Geometry: final body of the model. Coordinates: model frame, mm. Face numbers are marked on the shaded views. A direction names the side the tool comes from. Round coordinates to 2 decimals unless told otherwise and drop trailing zeros. Order: outer loops, then holes, each group sorted by start corner. A loop starts at its lowest first (then second) coordinate and runs counter-clockwise, first axis right, second up. Notation, with made-up numbers: M 61.5,58.25 L 65.5,58.25 A13 ccw 65.5,67.25 Z; hole C 10.25,67 d5. An arc over 180 degrees is marked long. Return JSON: item names as keys, results as strings. Group by question number.
Q1. Cut plane A-A on y = 3.5. Output: boundary loops of the cut face in (x, z), and give its area (3 significant figures).
Q2. Access query for the marked faces 1 and 2. Directions: +Z, -Z, +X, -X, +Y, -Y. A direction counts if a zero-diameter tool reaches every point of the face in a straight line with its end or side. Return the directions, or none.
Q3. Cut plane B-B on x = -50. Output: boundary loops of the cut face in (y, z).
Q4. Mould query, pull axis X, two halves, no side actions, for the marked faces 3, 4 and 5. Classes: released by +X, released by -X, zero draft, split by the parting line, or undercut.
Q5. Cut plane D-D on x = 67. Output: boundary loops of the cut face in (y, z), and give its area (3 significant figures).
Q6. Contact query for flat-ended pins moving along their axis: pin 1 (4 mm diameter, centred on x = -67, y = 10, fed in from -Z); pin 2 (6 mm diameter, centred on x = 0, y = 6, fed in from -Z); pin 3 (6 mm diameter, centred on y = 16, z = -4, fed in from -X). Output: stop coordinate, or through.
Q7. Cut plane C-C on z = -3. Output: boundary loops of the cut face in (x, y).
Q8. Ray query, probe 1 along X at (y, z) = (10, -7.75); probe 2 along Y at (x, z) = (-67, 5.75); probe 3 along X at (y, z) = (12, -6). Return the intervals inside material, ascending.
```python
from build123d import *

# Parameters (mm, degrees)
SKETCH1_W           = 150
SKETCH1_H           = 20
SKETCH1_R           = 4.05
BOSS_EXTRUDE1_DEPTH = 20
FILLET1_R           = 10
SKETCH3_R           = 1.55
CUT_EXTRUDE1_DEPTH  = 81.156097709
SKETCH3_3_R         = 3.5
SKETCH3_3_R_2       = 1.55
CUT_EXTRUDE2_DEPTH  = 3
CUT_EXTRUDE3_DEPTH  = 79.262379347
FILLET2_R           = 12


with BuildPart() as part:
    # Sketch1 → Boss-Extrude1 (new body)
    with BuildSketch(Plane(origin=(0, 0, 0), x_dir=(1, 0, 0), z_dir=(0, 1, 0))):
        Rectangle(SKETCH1_W, SKETCH1_H)
        with Locations(Location((-25, 3, 0), (0, 0, 270))):
            Circle(SKETCH1_R, mode=Mode.SUBTRACT)
        with Locations(Location((25, 3, 0), (0, 0, 270))):
            Circle(SKETCH1_R, mode=Mode.SUBTRACT)
        with Locations(Location((-50, 3, 0), (0, 0, 270))):
            Circle(SKETCH1_R, mode=Mode.SUBTRACT)
        with Locations(Location((50, 3, 0), (0, 0, 270))):
            Circle(SKETCH1_R, mode=Mode.SUBTRACT)
    extrude(amount=BOSS_EXTRUDE1_DEPTH)

    # Fillet1
    fillet1_edges = [part.edges().sort_by_distance(p)[0] for p in [
        (-75, 10, -10),
        (75, 10, -10),
    ]]
    fillet(fillet1_edges, radius=FILLET1_R)

    # Sketch3 → Cut-Extrude1 (cut, through all)
    with BuildSketch(Plane(origin=(0, 0, -10), x_dir=(-1, 0, 0), z_dir=(0, 0, -1))):
        with Locations((-67, 10)):
            Circle(SKETCH3_R)
        with Locations((67, 10)):
            Circle(SKETCH3_R)
    extrude(amount=-CUT_EXTRUDE1_DEPTH, mode=Mode.SUBTRACT)

    # Sketch3_3 → Cut-Extrude2 (cut)
    # profile 1 of 2: a face of its own
    with BuildSketch(Plane(origin=(0, 0, -10), x_dir=(-1, 0, 0), z_dir=(0, 0, -1))):
        with Locations((-67, 10)):
            Circle(SKETCH3_3_R)
        with Locations((-67, 10)):
            Circle(SKETCH3_3_R_2, mode=Mode.SUBTRACT)
    # profile 2 of 2: a face of its own
    with BuildSketch(Plane(origin=(0, 0, -10), x_dir=(-1, 0, 0), z_dir=(0, 0, -1))):
        with Locations((67, 10)):
            Circle(SKETCH3_3_R)
        with Locations((67, 10)):
            Circle(SKETCH3_3_R_2, mode=Mode.SUBTRACT)
    extrude(amount=-CUT_EXTRUDE2_DEPTH, mode=Mode.SUBTRACT)

    # Sketch4 → Cut-Extrude3 (cut, through all)
    with BuildSketch(Plane(origin=(0, 20, 0), x_dir=(1, 0, 0), z_dir=(0, 1, 0))):
        with BuildLine():
            Line((-6, 20), (6, 20))
            ThreePointArc((6, 20), (16, 10), (6, 0))
            Line((6, 0), (-6, 0))
            ThreePointArc((-6, 0), (-16, 10), (-6, 20))
        make_face()
    extrude(amount=-CUT_EXTRUDE3_DEPTH, mode=Mode.SUBTRACT)

    # Fillet2
    fillet2_edges = [part.edges().sort_by_distance(p)[0] for p in [
        (16, 10, -10),
        (-16, 10, -10),
    ]]
    fillet(fillet2_edges, radius=FILLET2_R)


solid = part.part
```
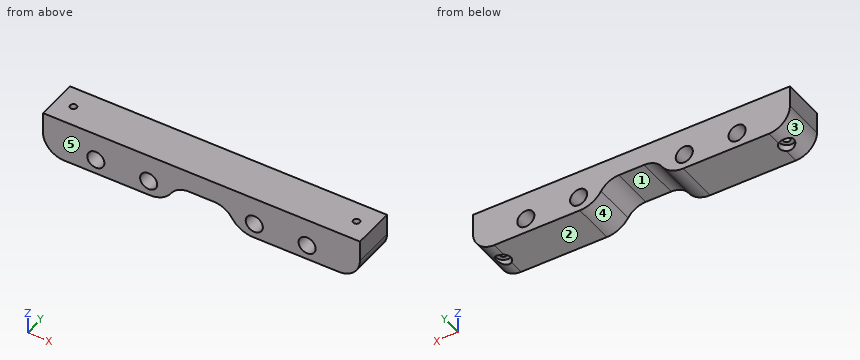
Result sheet:
{
 "1": {"outline": "M -75,0 A10 ccw -65,-10 L -24.44,-10 A12 ccw -14.38,-4.55 A10 cw -6,0 L 6,0 A10 cw 14.38,-4.55 A12 ccw 24.44,-10 L 65,-10 A10 ccw 75,0 L 75,10 L -75,10 Z; hole C -50,-3 d8.1; hole C -25,-3 d8.1; hole C 25,-3 d8.1; hole C 50,-3 d8.1", "area": "2,450 mm²"},
 "2": {"face 1": "-Z, +Y, -Y", "face 2": "-Z, +X, -X, +Y, -Y"},
 "3": {"outline": "M 0,-10 L 20,-10 L 20,-7.05 L 0,-7.05 Z; M 0,1.05 L 20,1.05 L 20,10 L 0,10 Z"},
 "4": {"face 3": "released by -X", "face 4": "undercut", "face 5": "zero draft"},
 "5": {"outline": "M 0,-9.8 L 6.5,-9.8 L 6.5,-7 L 8.45,-7 L 8.45,10 L 0,10 Z; M 11.55,-7 L 13.5,-7 L 13.5,-9.8 L 20,-9.8 L 20,10 L 11.55,10 Z", "area": "324 mm²"},
 "6": {"pin 1": "stops at z = -7", "pin 2": "stops at z = 0", "pin 3": "stops at x = -74.95"},
 "7": {"outline": "M -74.54,0 L -54.05,0 L -54.05,20 L -74.54,20 Z; M -45.95,0 L -29.05,0 L -29.05,20 L -45.95,20 Z; M -20.95,0 L -13.14,0 L -13.14,20 L -20.95,20 Z; M 13.14,0 L 20.95,0 L 20.95,20 L 13.14,20 Z; M 29.05,0 L 45.95,0 L 45.95,20 L 29.05,20 Z; M 54.05,0 L 74.54,0 L 74.54,20 L 54.05,20 Z; hole C -67,10 d3.1; hole C 67,10 d3.1"},
 "8": {"probe 1": "x = -71.32 to -70.5, -63.5 to -17.44, 17.44 to 63.5, 70.5 to 71.32", "probe 2": "y = 0 to 8.45, 11.55 to 20", "probe 3": "x = -73 to -52.72, -47.28 to -27.72, -22.28 to -15.49, 15.49 to 22.28, 27.72 to 47.28, 52.72 to 73"}
}
